Can you work these out from the model? Positions are in its coordinate system, mm. Give positions to 0.01 mm unless a question says otherwise; leave off trailing zeros. Loops run counter-clockwise (first coordinate to the right, second up) from the corner with the lowest first, then second, coordinate; pieces in that order, holes last. Notation, with made-up numbers: M 60.25,0.25 L 103.25,0.25 A3 cw 103.25,5.25 Z; hole C 48.5,84.25 d4. An arc over 180 degrees is marked long. Put each result on its own line as item: value. Start each with the question number.
1) Please list where these lines run through material, in increasing order: line 1 along Y through (x, z) = (5.5, 1); line 2 along Y through (x, z) = (-0.5, 4.75); line 3 along X through (y, z) = (104.5, 4.25). Write a range as from..to.
2) For P1, Ø7, axis at x = 3, y = 129.02, coming from the +Z side; P2, Ø4, axis at x = 3, y = 78.22, coming from the +Z side; P3, Ø5.5, axis at x = 4.5, y = 147.5, coming from the +Z side, each with a flat end and sliding along its axis, tell me the tip position at first contact or that it passes through.
3) Imagine slicing it at A-A (z = 5.5). Write out the boundary of the cut face in (x, y), then the cut area to 3 significant figures.
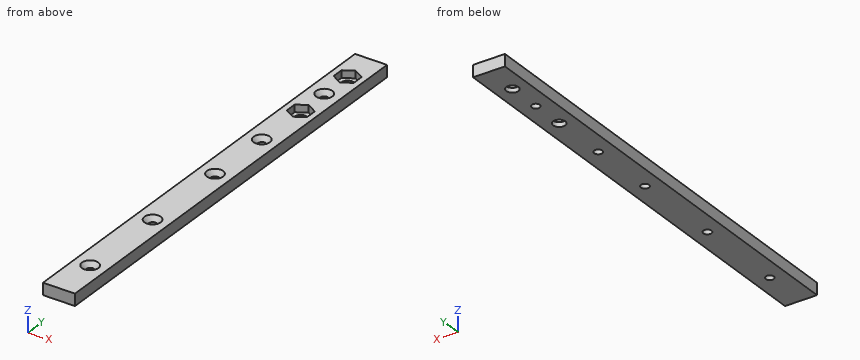
from build123d import *

# Parameters (mm, degrees)
F0_W           = 17.78
F0_H           = 254
F1_DEPTH       = 6.604
F0_R           = 3.3782
F2_DEPTH       = 2.54
F4_D           = 4.4958
F4_CSINK_D     = 9.1186
F4_CSINK_ANGLE = 82


with BuildPart() as f1:
    # F0 (on Top) → F1 (new body)
    with BuildSketch(Plane.XY):
        with Locations((3.0019969136, 40.122719574)):
            Rectangle(F0_W, F0_H)
        Polygon((8.5899969136, 113.1989528782), (8.5899969136, 106.7464862697), (3.0019969136, 103.5202529655), (-2.5860030864, 106.7464862697), (-2.5860030864, 113.1989528782), (3.0019969136, 116.4251861824), align=None, mode=Mode.SUBTRACT)
        Polygon((3.0019969136, 154.5251861824), (8.5899969136, 151.2989528782), (8.5899969136, 144.8464862697), (3.0019969136, 141.6202529655), (-2.5860030864, 144.8464862697), (-2.5860030864, 151.2989528782), align=None, mode=Mode.SUBTRACT)
    extrude(amount=F1_DEPTH)

    # F0 (on Top) → F2 (join)
    with BuildSketch(Plane.XY):
        Polygon((3.0019969136, 103.5202529655), (8.5899969136, 106.7464862697), (8.5899969136, 113.1989528782), (3.0019969136, 116.4251861824), (-2.5860030864, 113.1989528782), (-2.5860030864, 106.7464862697), align=None)
        with Locations((3.0019969136, 109.972719574)):
            Circle(F0_R, mode=Mode.SUBTRACT)
        Polygon((8.5899969136, 144.8464862697), (8.5899969136, 151.2989528782), (3.0019969136, 154.5251861824), (-2.5860030864, 151.2989528782), (-2.5860030864, 144.8464862697), (3.0019969136, 141.6202529655), align=None)
        with Locations((3.0019969136, 148.072719574)):
            Circle(F0_R, mode=Mode.SUBTRACT)
    extrude(amount=F2_DEPTH)

    # F4 (through all)
    with Locations(Plane.XY.offset(6.604)):
        with Locations((3.0019969136, 129.022719574), (3.0019969136, 78.222719574), (3.0019969136, 40.122719574), (3.0019969136, -10.677280426), (3.0019969136, -61.477280426)):
            CounterSinkHole(F4_D / 2, F4_CSINK_D / 2, counter_sink_angle=F4_CSINK_ANGLE)


solid = f1.part
Recorded:
1. line 1: -86.88..107.7, 112.25..145.8, 150.35..167.12
1. line 2: -86.88..105.54, 114.4..143.64, 152.5..167.12
1. line 3: -5.89..1.31, 4.7..11.89
2. P1: z = 5.39
2. P2: through
2. P3: z = 2.54
3. outline: M -5.89,-86.88 L 11.89,-86.88 L 11.89,167.12 L -5.89,167.12 Z; hole M -2.59,106.75 L 3,103.52 L 8.59,106.75 L 8.59,113.2 L 3,116.43 L -2.59,113.2 Z; hole M -2.59,144.85 L 3,141.62 L 8.59,144.85 L 8.59,151.3 L 3,154.53 L -2.59,151.3 Z; hole C 3,-61.48 d7.2; hole C 3,-10.68 d7.2; hole C 3,40.12 d7.2; hole C 3,78.22 d7.2; hole C 3,129.02 d7.2
3. area: 4,100 mm²
